Verification items for the finished model (mm, model axes). Give positions to 0.01 mm unless a question says otherwise; leave off trailing zeros. Write each loop counter-clockwise with the first axis right and the second up, starting at its lowest first coordinate (ties: lowest second). Pieces come first, ordered by that corner, then holes.
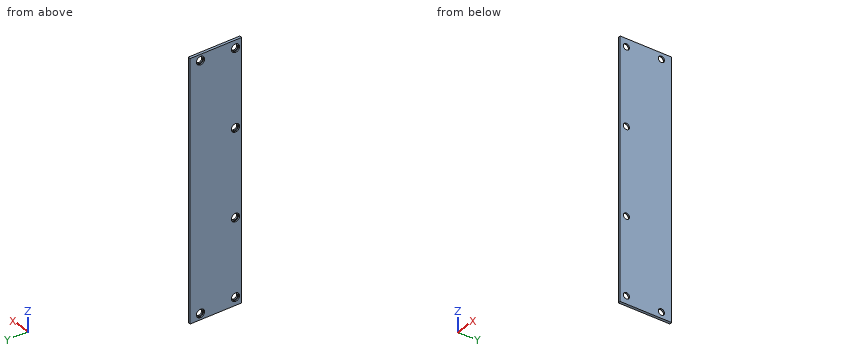
from build123d import *

# Parameters (mm, degrees)
SKETCH3_W           = 1.27
SKETCH3_H           = 25.4
BOSS_EXTRUDE1_DEPTH = 127
SKETCH5_R           = 1.524
CUT_EXTRUDE1_DEPTH  = 1.27
SKETCH6_R           = 2.032
SKETCH6_R_2         = 1.524
CUT_EXTRUDE3_DEPTH  = 0.635


with BuildPart() as part:
    # Sketch3 → Boss-Extrude1 (new body)
    with BuildSketch(Plane.XY):
        with Locations((0, -12.7)):
            Rectangle(SKETCH3_W, SKETCH3_H)
    extrude(amount=-BOSS_EXTRUDE1_DEPTH)

    # Sketch5 → Cut-Extrude1 (cut)
    with BuildSketch(Plane.ZY.offset(0.635)):
        with Locations(Location((-123.063, -22.352, 0), (0, 0, 270))):
            Circle(SKETCH5_R)
        with Locations(Location((-84.963, -22.352, 0), (0, 0, 270))):
            Circle(SKETCH5_R)
        with Locations(Location((-123.952, -5.08, 0), (0, 0, 270))):
            Circle(SKETCH5_R)
        with Locations(Location((-42.037, -22.352, 0), (0, 0, 90))):
            Circle(SKETCH5_R)
        with Locations(Location((-3.937, -22.352, 0), (0, 0, 90))):
            Circle(SKETCH5_R)
        with Locations(Location((-3.048, -5.08, 0), (0, 0, 90))):
            Circle(SKETCH5_R)
    extrude(amount=-CUT_EXTRUDE1_DEPTH, mode=Mode.SUBTRACT)

    # Sketch6 → Cut-Extrude3 (cut)
    # profile 1 of 6: a face of its own
    with BuildSketch(Plane.ZY.offset(0.635)):
        with Locations(Location((-123.063, -22.352, 0), (0, 0, 270))):
            Circle(SKETCH6_R)
        with Locations(Location((-123.063, -22.352, 0), (0, 0, 270))):
            Circle(SKETCH6_R_2, mode=Mode.SUBTRACT)
    # profile 2 of 6: a face of its own
    with BuildSketch(Plane.ZY.offset(0.635)):
        with Locations(Location((-84.963, -22.352, 0), (0, 0, 270))):
            Circle(SKETCH6_R)
        with Locations(Location((-84.963, -22.352, 0), (0, 0, 270))):
            Circle(SKETCH6_R_2, mode=Mode.SUBTRACT)
    # profile 3 of 6: a face of its own
    with BuildSketch(Plane.ZY.offset(0.635)):
        with Locations(Location((-42.037, -22.352, 0), (0, 0, 270))):
            Circle(SKETCH6_R)
        with Locations(Location((-42.037, -22.352, 0), (0, 0, 270))):
            Circle(SKETCH6_R_2, mode=Mode.SUBTRACT)
    # profile 4 of 6: a face of its own
    with BuildSketch(Plane.ZY.offset(0.635)):
        with Locations(Location((-3.937, -22.352, 0), (0, 0, 270))):
            Circle(SKETCH6_R)
        with Locations(Location((-3.937, -22.352, 0), (0, 0, 270))):
            Circle(SKETCH6_R_2, mode=Mode.SUBTRACT)
    # profile 5 of 6: a face of its own
    with BuildSketch(Plane.ZY.offset(0.635)):
        with Locations(Location((-3.048, -5.08, 0), (0, 0, 270))):
            Circle(SKETCH6_R)
        with Locations(Location((-3.048, -5.08, 0), (0, 0, 270))):
            Circle(SKETCH6_R_2, mode=Mode.SUBTRACT)
    # profile 6 of 6: a face of its own
    with BuildSketch(Plane.ZY.offset(0.635)):
        with Locations(Location((-123.952, -5.08, 0), (0, 0, 270))):
            Circle(SKETCH6_R)
    extrude(amount=-CUT_EXTRUDE3_DEPTH, mode=Mode.SUBTRACT)


solid = part.part
Item 1: Sectioned sample at B-B on y = -22.75. State how many separate pieces and enclosed holes the cut face has, then the cut area to 3 significant figures.
Answer key:
separate pieces: 5
enclosed holes: 0
area: 144 mm2
Item 2: Scan lines: line 1 along Z through (x, y) = (0.45, -5.08); line 2 along Z through (x, y) = (-0.15, -22.25); line 3 along Z through (x, y) = (-0.15, -5). Record each from-to range of solid material in increasing order.
Answer key:
line 1: z = -127 to -125.48, -122.43 to -4.57, -1.52 to 0
line 2: z = -127 to -125.09, -121.03 to -86.99, -82.93 to -44.07, -40.01 to -5.97, -1.91 to 0
line 3: z = -127 to -125.98, -121.92 to -5.08, -1.02 to 0
Item 3: Sectioned sample at A-A on y = -5.08. Record the cut outline in (x, z) (3 decimals).
Answer key:
outline: (-0.635, -127) - (0.635, -127) - (0.635, -125.476) - (0, -125.476) - (0, -125.984) - (-0.635, -125.984) - close; (-0.635, -121.92) - (0, -121.92) - (0, -122.428) - (0.635, -122.428) - (0.635, -4.572) - (0, -4.572) - (0, -5.08) - (-0.635, -5.08) - close; (-0.635, -1.016) - (0, -1.016) - (0, -1.524) - (0.635, -1.524) - (0.635, 0) - (-0.635, 0) - close
Item 4: Depth check by flat-ended pin: pin 1 (1.2 mm diameter, centred on y = -5.5, z = -123, fed in from -X); pin 2 (1.2 mm diameter, centred on y = -22, z = -84.5, fed in from -X). Enter the tip coordinate at first touch or a pass-through.
Answer key:
pin 1: stops at x = 0
pin 2: passes through
